Geometry check sheet. Reference: the model listing, model coordinates, mm. A direction names the side the tool comes from. Round coordinates to 2 decimals unless told otherwise and drop trailing zeros. Answer as CSV lines item,"result". Start each with the question number.
Autodesk Inventor part; units mm, degrees
ref_plane "YZ Plane" through (0, 0, 0) normal (1, 0, 0) x (0, 1, 0)
ref_plane "XZ Plane" through (0, 0, 0) normal (0, 1, 0) x (-1, 0, 0)
ref_plane "XY Plane" through (0, 0, 0) normal (0, 0, 1) x (1, 0, 0)
sketch "Boceto1" plane through (0, 0, 0) normal (0, 0, 1) x (1, 0, 0)
  line L0 (0, 20) -> (7, 20)
  line L1 (7, 20) -> (7, 21)
  line L2 (0, 20) -> (1, 20)
  line L3 (1, 17.6407) -> (1, 15)
  line L4 (-1, 13) -> (0, 13)
  line L5 (5, 19) -> (2.3598, 19)
  arc A0 (5, 19) -> (6.7321, 20) centre (5, 21) ccw
  arc A1 (0, 13.2679) -> (1, 15) centre (-1, 15) ccw
  line L6 (20, 20) -> (13, 20)
  line L7 (19.3, 20) -> (19, 20)
  line L8 (19, 17.6402) -> (19, 15)
  line L9 (21, 13) -> (20, 13)
  line L10 (13, 20) -> (13, 21)
  line L11 (15, 19) -> (18.365, 19)
  arc A2 (13.2679, 20) -> (15, 19) centre (15, 21) ccw
  arc A3 (19, 15) -> (20, 13.2679) centre (21, 15) ccw
  line L12 (0.7, 0) -> (7, 0)
  line L13 (-1, 8.6378) -> (0, 8.6378)
  line L14 (7, 0) -> (7, -1)
  line L15 (5, 1) -> (2.3593, 1)
  line L16 (19.3, 0) -> (13, 0)
  line L17 (13, 0) -> (13, -1)
  line L18 (15, 1) -> (17.6402, 1)
  line L19 (19, 5) -> (19, 2.3593)
  arc A4 (20, 6.7321) -> (19, 5) centre (21, 5) ccw
  arc A5 (15, 1) -> (13.2679, 0) centre (15, -1) ccw
  arc A6 (6.7321, 0) -> (5, 1) centre (5, -1) ccw
  line L20 (20, 20) -> (13, 20)
  line L21 (7, 20) -> (0.7, 20)
  line L22 (0, 19.3) -> (0, 13)
  line L23 (0, 6.4641) -> (0, 0.7)
  line L24 (20, 0.7) -> (20, 6.7321)
  line L25 (20, 13) -> (20, 19.3)
  line L26 (0, 0) -> (7, 0)
  line L27 (13, 0) -> (20, 0)
  line L28 (17.6407, 19) -> (17.365, 19)
  line L29 (17.8529, 18.4879) -> (13.565, 14.2)
  line L30 (18.4883, 17.8528) -> (14.2, 13.5832)
  line L31 (1.5121, 17.8529) -> (5.8, 13.565)
  line L32 (2.1472, 18.4883) -> (6.4168, 14.2)
  line L33 (2.1471, 1.5121) -> (6.435, 5.8)
  line L34 (1.5117, 2.1472) -> (5.8, 6.4168)
  line L35 (18.4879, 2.1471) -> (14.2, 6.435)
  line L36 (17.8528, 1.5117) -> (13.5832, 5.8)
  line L37 (13, 13) -> (11.6766, 13.2679)
  line L38 (11.6766, 13.2679) -> (10.9786, 12.57)
  line L39 (13, 13) -> (13.2679, 11.6766)
  line L40 (13.2679, 11.6766) -> (12.57, 10.9786)
  line L41 (6.7321, 11.6766) -> (7.43, 10.9786)
  line L42 (7, 13) -> (6.7321, 11.6766)
  line L43 (7, 13) -> (8.3234, 13.2679)
  line L44 (8.3234, 13.2679) -> (9.0214, 12.57)
  line L45 (8.3234, 6.7321) -> (9.0214, 7.43)
  line L46 (7, 7) -> (8.3234, 6.7321)
  line L47 (7, 7) -> (6.7321, 8.3234)
  line L48 (6.7321, 8.3234) -> (7.43, 9.0214)
  line L49 (13.2679, 8.3234) -> (12.57, 9.0214)
  line L50 (13, 7) -> (13.2679, 8.3234)
  line L51 (13, 7) -> (11.6766, 6.7321)
  line L52 (11.6766, 6.7321) -> (10.9786, 7.43)
  line L53 (7, 13) -> (5.8, 14.2) construction
  line L54 (5.8, 5.8) -> (7, 7) construction
  line L55 (14.2, 5.8) -> (13, 7) construction
  line L56 (11.9445, 8.0555) -> (8.0555, 11.9445) construction
  line L57 (8.0555, 8.0555) -> (11.9445, 11.9445) construction
  line L58 (13, 13) -> (14.2, 14.2) construction
  arc A7 (10.9786, 12.57) -> (9.0214, 12.57) centre (10, 10) ccw
  arc A8 (12.57, 9.0214) -> (12.57, 10.9786) centre (10, 10) ccw
  arc A9 (7.43, 10.9786) -> (7.43, 9.0214) centre (10, 10) ccw
  arc A10 (9.0214, 7.43) -> (10.9786, 7.43) centre (10, 10) ccw
  line L59 (13.94, 10) -> (14.2, 10.9786)
  line L60 (13.94, 10) -> (14.2, 9.0214)
  line L61 (14.2, 6.435) -> (14.2, 9.0214)
  line L62 (14.2, 10.9786) -> (14.2, 13.5832)
  line L63 (10, 13.94) -> (10.9786, 14.2)
  line L64 (10.9786, 14.2) -> (10, 13.94)
  line L65 (10, 13.94) -> (9.0214, 14.2)
  line L66 (6.06, 10) -> (5.8, 10.9786)
  line L67 (6.06, 10) -> (5.8, 9.0214)
  line L68 (10, 6.06) -> (10.9786, 5.8)
  line L69 (10, 6.06) -> (9.0214, 5.8)
  line L70 (6.435, 5.8) -> (9.0214, 5.8)
  line L71 (10.9786, 5.8) -> (13.5832, 5.8)
  line L72 (5.8, 13.565) -> (5.8, 10.9786)
  line L73 (5.8, 9.0214) -> (5.8, 6.4168)
  line L74 (13.565, 14.2) -> (10.9786, 14.2)
  line L75 (9.0214, 14.2) -> (6.4168, 14.2)
  line L76 (1, 2.3598) -> (1, 4.7321)
  arc A11 (1, 4.7321) -> (0, 6.4641) centre (-1, 4.7321) ccw
  arc A12 (0.7, 20) -> (0, 19.3) centre (0.7, 19.3) ccw
  arc A13 (20, 19.3) -> (19.3, 20) centre (19.3, 19.3) ccw
  arc A14 (19.3, 0) -> (20, 0.7) centre (19.3, 0.7) ccw
  arc A15 (0, 0.7) -> (0.7, 0) centre (0.7, 0.7) ccw
  arc A16 (2.3598, 19) -> (2.1472, 18.4883) centre (2.3598, 18.7) ccw
  arc A17 (1.5121, 17.8529) -> (1, 17.6407) centre (1.3, 17.6407) ccw
  arc A18 (17.8529, 18.4879) -> (17.6407, 19) centre (17.6407, 18.7) ccw
  arc A19 (19, 17.6402) -> (18.4883, 17.8528) centre (18.7, 17.6402) ccw
  arc A20 (18.4879, 2.1471) -> (19, 2.3593) centre (18.7, 2.3593) ccw
  arc A21 (17.6402, 1) -> (17.8528, 1.5117) centre (17.6402, 1.3) ccw
  arc A22 (2.1471, 1.5121) -> (2.3593, 1) centre (2.3593, 1.3) ccw
  arc A23 (1, 2.3598) -> (1.5117, 2.1472) centre (1.3, 2.3598) ccw
  point P0 (7, 19)
  point P1 (1, 13)
  point P2 (19, 13)
  point P3 (1, 1.6378)
  point P4 (1, 8.6378)
  point P5 (7, 1)
  point P6 (13, 1)
  point P7 (19, 1.635)
  point P8 (1, 18.365)
  point P9 (19, 18.3622)
  point P10 (19.6406, 19)
  point P11 (1, 19.6406)
  point P12 (0.3594, 1)
  point P13 (19, 0.3594)
  point P14 (1.6378, 19)
  point P15 (1.635, 1)
  point P16 (18.3622, 1)
  dimension "d1" = 20
  dimension "d2" = 20
  dimension "d5" = 7
  dimension "d6" = 1
  dimension "d7" = 1
  dimension "d8" = 7
  dimension "d9" = 2
  dimension "d10" = 2
  dimension "d11" = 7
  dimension "d12" = 1
  dimension "d13" = 7
  dimension "d14" = 2
  dimension "d15" = 7
  dimension "d16" = 1
  dimension "d17" = 7
  dimension "d20" = 8.4
  dimension "d21" = 8.4
  dimension "d23" = 0.9
  dimension "d26" = 360
  dimension "d30" = 360
  dimension "d38" = 2
  dimension "d41" = 0.7
  dimension "d42" = 0.3
extrude "Extrusión3" add sketch "Boceto1" against normal blind 146
properties part number "PerfilBaseJohan"
1. Access from +Z, -Z, +X, -X, +Y, -Y to the whole of each face (thin tool, end or side, straight path). Record for faces 1 (the face through (4, 20, -72)), 2 (the face through (19, 4, -72)).
2. Thickness scan on probe 1 along Y at (x, z) = (18.5, -69.5); probe 2 along Y at (x, z) = (6.25, -28.5) (3 decimals); probe 3 along Y at (x, z) = (11, -88). Record the ranges inside material, lowest first.
3. Go/stop test with flat-tipped pins: pin 1 Ø0.8 at (y, z) = (12, -85) entering from -X; pin 2 Ø1.3 at (x, z) = (12, -102.5) entering from +Y; pin 3 Ø1.3 at (y, z) = (12.5, -88.5) entering from +X. Record where each tip stops, or that it passes through.
4. Draft check along X on faces 3 (the face through (0, 4, -72)), 4 (the face through (4, 19, -72)), 5 (the face through (4, 0, -72)). Enter one of: released by +X, released by -X, zero draft, split by the parting line, or undercut.
Numbers:
1,face 1,"+Z, -Z, +X, -X, +Y"
1,face 2,"+Z, -Z"
2,probe 1,"y = 0 to 2.14, 17.86 to 20"
2,probe 2,"y = 0 to 0.561, 5.615 to 14.368, 19.439 to 20"
2,probe 3,"y = 5.8 to 7.41, 12.59 to 14.2"
3,pin 1,"stops at x = 5.8"
3,pin 2,"stops at y = 14.2"
3,pin 3,"stops at x = 14.2"
4,face 3,"released by -X"
4,face 4,"undercut"
4,face 5,"zero draft"
